Autodesk Inventor part; units mm, degrees
ref_plane "YZ Plane" through (0, 0, 0) normal (1, 0, 0) x (0, 1, 0)
ref_plane "XZ Plane" through (0, 0, 0) normal (0, 1, 0) x (-1, 0, 0)
ref_plane "XY Plane" through (0, 0, 0) normal (0, 0, 1) x (1, 0, 0)
sketch "Sketch1" plane through (0, 0, 0) normal (0, 0, 1) x (1, 0, 0)
  circle A0 centre (0, 0) radius 17.5
  circle A1 centre (0, 0) radius 10
  dimension "d0" = 35
  dimension "d1" = 20
extrude "Extrusion1" add sketch "Sketch1" along normal blind 4
fillet "Fillet1" radius 2 2 edges at (-17.5, 0, 4) (-17.5, 0, 0)
fillet "Fillet2" radius 1 2 edges at (-10, 0, 0) (-10, 0, 4)
properties part number "Thrust Bearing" material "Stainless Steel"
Part model, mm, in its own coordinate system. Round coordinates to 2 decimals unless told otherwise and drop trailing zeros. Loops run counter-clockwise (first coordinate to the right, second up) from the corner with the lowest first, then second, coordinate; pieces in that order, holes last.
Item 1: Drop flat-ended pins along their axis: P1, Ø2, axis at x = 0, z = 3.5, coming from the -Y side; P2, Ø1, axis at y = 12.5, z = 2, coming from the -X side; P3, Ø3, axis at x = 8, y = 4.5, coming from the +Z side. Give the stop position or say it passes through.
Item 2: Mould opens along X. For faces 1 (the face through (-2.17, 9.76, 1.99)), 2 (the face through (-11, -3, 0)) say: +X half, -X half, draft (parallel to the pull), parting line (faces both ways), or undercut.
Item 3: Drill centre lines: line 1 (X direction, y = 9, z = 2.1); line 2 (X direction, y = -8.5, z = 3.7); line 3 (Y direction, x = 8.5, z = 2). Where is each one in solid material? Low to high.
Item 4: Cut at C-C, the plane z = 3.5. Give the cut face in (x, y).
A:
1. P1: stops at y = -17.44
1. P2: stops at x = -12.74
1. P3: stops at z = 3.95
2. face 1: undercut
2. face 2: draft
3. line 1: x = -15.01 to -4.36, 4.36 to 15.01
3. line 2: x = -14.21 to -5.79, 5.79 to 14.21
3. line 3: y = -15.3 to -5.27, 5.27 to 15.3
4. outline: circle Ø33.65 at (0, 0); hole circle Ø20.27 at (0, 0)
